Read the model definition and answer for the solid it produces. Units are mm, in the model's axes. Face numbers are marked on the shaded views. Round coordinates to 2 decimals unless told otherwise and drop trailing zeros. Order: outer loops, then holes, each group sorted by start corner. A loop starts at its lowest first (then second) coordinate and runs counter-clockwise, first axis right, second up. Notation, with made-up numbers: M -11,19.5 L 3,19.5 A16 ccw 3,32.5 Z; hole C 11.25,-28 d8. An arc over 180 degrees is marked long. Answer as CSV lines item,"result".
```python
from build123d import *

# Parameters (mm, degrees)
F0_W     = 14.732
F0_H     = 7.112
F0_R     = 2.0066
F0_R_2   = 2.6924
F1_DEPTH = 25.4
F2_DEPTH = 25.401
F3_DEPTH = 4.064
F4_R     = 1.3208
F5_DEPTH = 25.401
F6_R     = 0.762
F7_R     = 3.175


# Not quite as in the source:
# - a feature names something its author has since deleted; it is built from what else it names


with BuildPart() as f1:
    # F0 (on Front) → F1 (new body)
    with BuildSketch(Plane.XZ):
        Rectangle(F0_W, F0_H)
        with Locations((-4.699, 0)):
            Circle(F0_R, mode=Mode.SUBTRACT)
        with Locations((3.302, 0)):
            Circle(F0_R_2, mode=Mode.SUBTRACT)
        with Locations((3.302, 0)):
            Circle(F0_R_2)
        with Locations((-4.699, 0)):
            Circle(F0_R)
    extrude(amount=F1_DEPTH)

    # F0 (on Front) → F2 (cut, through all)
    with BuildSketch(Plane.XZ):
        with Locations((3.302, 0)):
            Circle(F0_R_2)
    extrude(amount=F2_DEPTH, mode=Mode.SUBTRACT)

    # F0 (on Front) → F3 (join)
    with BuildSketch(Plane.XZ):
        with Locations((-4.699, 0)):
            Circle(F0_R)
    extrude(amount=-F3_DEPTH)

    # F4 (on face) → F5 (cut, through all)
    with BuildSketch(Plane.XZ):
        with Locations((3.302, 0)):
            Circle(F4_R)
    extrude(amount=F5_DEPTH, mode=Mode.SUBTRACT)

    # F6
    f6_edges = [f1.edges().sort_by_distance(p)[0] for p in [
        (-6.7056, 4.064, 0),
    ]]
    fillet(f6_edges, radius=F6_R)

    # F7
    f7_edges = [f1.edges().sort_by_distance(p)[0] for p in [
        (7.366, -12.7, 3.556),
        (7.366, -12.7, -3.556),
        (-7.366, -12.7, -3.556),
        (-7.366, -12.7, 3.556),
    ]]
    fillet(f7_edges, radius=F7_R)


solid = f1.part
```
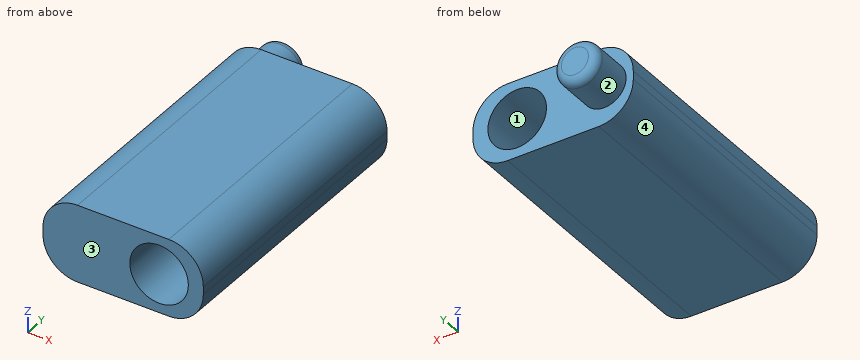
Item 1: A cutting plane is placed at C-C, the plane x = 3. Determine the outline of the cut face in (y, z).
Ans:
outline,"M -25.4,-3.56 L 0,-3.56 L 0,-2.68 L -25.4,-2.68 Z; M -25.4,2.68 L 0,2.68 L 0,3.56 L -25.4,3.56 Z"
Item 2: Flat-ended cylindrical pins translate along their axes: pin 1 (4 mm diameter, centred on x = 1, z = 1.5, fed in from +Y); pin 2 (3 mm diameter, centred on x = 4, z = -2.5, fed in from -Y). Find the tip coordinate at first contact, or state that the pin passes through.
Ans:
pin 1,"y = 0"
pin 2,"y = -25.4"
Item 3: A cutting plane is placed at D-D, the plane x = -1.5. Determine the outline of the cut face in (y, z).
Ans:
outline,"M -25.4,-3.56 L 0,-3.56 L 0,3.56 L -25.4,3.56 Z"
Item 4: Determine the mould class of the marked faces 1, 2, 3 and 4 for opening direction Z: +Z half, -Z half, draft (parallel to the pull), parting line (faces both ways), or undercut.
Ans:
face 1,"undercut"
face 2,"parting line"
face 3,"draft"
face 4,"-Z half"
Item 5: A cutting plane is placed at A-A, the plane y = -8. Determine the outline of the cut face in (x, z) (3 decimals).
Ans:
outline,"M -7.366,-0.381 A3.175 ccw -4.191,-3.556 L 4.191,-3.556 A3.175 ccw 7.366,-0.381 L 7.366,0.381 A3.175 ccw 4.191,3.556 L -4.191,3.556 A3.175 ccw -7.366,0.381 Z; hole C 3.302,0 d5.385"
Item 6: Find the intervals of material crossed by probe 1 along X at (y, z) = (-6.75, 0); probe 2 along Z at (x, y) = (1.5, -7.5); probe 3 along Y at (x, z) = (6.75, -0.25), in increasing order. Write a range as [from, to].
Ans:
probe 1,"[-7.37, 0.61], [5.99, 7.37]"
probe 2,"[-3.56, -2], [2, 3.56]"
probe 3,"[-25.4, 0]"
Item 7: A cutting plane is placed at B-B, the plane z = 0. Determine the outline of the cut face in (x, y).
Ans:
outline,"M -7.37,-25.4 L 0.61,-25.4 L 0.61,0 L -2.69,0 L -2.69,3.3 A0.76 ccw -3.45,4.06 L -5.94,4.06 A0.76 ccw -6.71,3.3 L -6.71,0 L -7.37,0 Z; M 5.99,-25.4 L 7.37,-25.4 L 7.37,0 L 5.99,0 Z"
